The listing builds one solid part. Answer for the finished solid, in the listing's coordinates (mm). A direction names the side the tool comes from. Give positions to 0.01 mm unless a question says otherwise; leave off trailing zeros. Order: outer loops, then holes, each group sorted by start corner. A loop starts at its lowest first (then second) coordinate and runs counter-clockwise, first axis right, second up.
```python
from build123d import *

# Parameters (mm, degrees)
SKETCH_1_R          = 54
SKETCH_1_R_2        = 3
EXTRUDE_1_DEPTH     = 5
SKETCH_3_R          = 4
CUT_EXTRUDE_2_DEPTH = 77.531039455
SKETCH_4_R          = 2
EXTRUDE_2_DEPTH     = 12
CUT_EXTRUDE_START   = -3.2
SKETCH_6_R          = 2
SKETCH_6_R_2        = 1.8
CUT_EXTRUDE_3_DEPTH = 0.5
SKETCH_7_R          = 4
EXTRUDE_3_DEPTH     = 2
CHAMFER_1_SIZE      = 1
CUT_EXTRUDE_START_2 = -0.5
SKETCH_9_W          = 2
SKETCH_9_H          = 2
CUT_EXTRUDE_5_DEPTH = 4
FILLET_1_R          = 0.1


with BuildPart() as part:
    # Sketch 1 → Extrude 1 (new body)
    with BuildSketch(Plane.XY):
        Circle(SKETCH_1_R)
        Circle(SKETCH_1_R_2, mode=Mode.SUBTRACT)
    extrude(amount=EXTRUDE_1_DEPTH)

    # Sketch 3 → Cut-Extrude 2 (cut, through all)
    with BuildSketch(Plane(origin=(0, 0, 0), x_dir=(-1, 0, 0), z_dir=(0, 0, -1))):
        with Locations((-5.091227954, 19.341132281)):
            Circle(SKETCH_3_R)
        with Locations((10.076203981, 17.276287603)):
            Circle(SKETCH_3_R)
        with Locations((19.341132281, 5.091227954)):
            Circle(SKETCH_3_R)
        with Locations((17.276287603, -10.076203981)):
            Circle(SKETCH_3_R)
        with Locations((5.091227954, -19.341132281)):
            Circle(SKETCH_3_R)
        with Locations((-10.076203981, -17.276287603)):
            Circle(SKETCH_3_R)
        with Locations((-19.341132281, -5.091227954)):
            Circle(SKETCH_3_R)
        with Locations((-17.276287603, 10.076203981)):
            Circle(SKETCH_3_R)
    extrude(amount=-CUT_EXTRUDE_2_DEPTH, mode=Mode.SUBTRACT)

    # Sketch 4 → Extrude 2 (add)
    with BuildSketch(Plane.XY.offset(5)):
        with Locations((2.976659474, 6.884003078)):
            Circle(SKETCH_4_R)
        with Locations((9.178670771, -3.968879298)):
            Circle(SKETCH_4_R)
    extrude(amount=EXTRUDE_2_DEPTH)

    # Sketch 6 → Cut-Extrude 3 (cut)
    with BuildSketch(Plane.XY.offset(17).offset(CUT_EXTRUDE_START)):
        with Locations((2.976659474, 6.884003078)):
            Circle(SKETCH_6_R)
        with Locations((2.976659474, 6.884003078)):
            Circle(SKETCH_6_R_2, mode=Mode.SUBTRACT)
    extrude(amount=CUT_EXTRUDE_3_DEPTH, mode=Mode.SUBTRACT)

    # Sketch 7 → Extrude 3 (add)
    with BuildSketch(Plane.XY.offset(17)):
        with Locations((9.178670771, -3.968879298)):
            Circle(SKETCH_7_R)
    extrude(amount=-EXTRUDE_3_DEPTH)

    # Chamfer 1
    chamfer_1_edges = [part.edges().sort_by_distance(p)[0] for p in [
        (0.976659474, 6.884003078, 5),
        (7.178670771, -3.968879298, 5),
    ]]
    chamfer(chamfer_1_edges, length=CHAMFER_1_SIZE)

    # Sketch 9 → Cut-Extrude 5 (cut)
    with BuildSketch(Plane.XY.offset(5).offset(CUT_EXTRUDE_START_2)):
        with Locations((0, -3)):
            Rectangle(SKETCH_9_W, SKETCH_9_H)
    extrude(amount=-CUT_EXTRUDE_5_DEPTH, mode=Mode.SUBTRACT)

    # Fillet 1
    fillet_1_edges = [part.edges().sort_by_distance(p)[0] for p in [
        (1, -4, 2.5),
        (-1, -4, 2.5),
    ]]
    fillet(fillet_1_edges, radius=FILLET_1_R)


solid = part.part
```
1) Find section B-B (z = 10.5). Write down the section's boundary in (x, y).
Geometry says:
outline: circle Ø4 at (2.98, 6.88); circle Ø4 at (9.18, -3.97)
2) Given P1, Ø8, axis at y = 16.5, z = 14.5, coming from the +X side; P2, Ø13, axis at x = -17.28, y = -10.08, coming from the +Z side; P3, Ø10, axis at y = -26.5, z = 4, coming from the -X side; P4, Ø0.5, axis at y = -3.5, z = 3.5, coming from the +X side, each flat-ended and moving along its own axis, determine where each tip first touches the part or whether it passes through.
Geometry says:
P1: passes through
P2: stops at z = 5
P3: stops at x = -49.54
P4: stops at x = 53.9
3) Find section A-A (z = 2.5). Count the separate pieces of the cut face and the enclosed holes in it, then the cut area to 3 significant figures.
Geometry says:
separate pieces: 1
enclosed holes: 9
area: 8,730 mm2
4) Find section D-D (y = -35). Write down the section's boundary in (x, z), then the cut area to 3 significant figures.
Geometry says:
outline: (-41.12, 0) - (41.12, 0) - (41.12, 5) - (-41.12, 5) - close
area: 411 mm2
5) A tool of negligible diameter and unlimited length cuts with its end or side. For faces 4 (the cylindrical face through (4.05, 8.57, 15.63)), 5 (the flat face through (9, -4, 17)), 6 (the cylindrical face through (7.18, -3.88, 10.44)), from which of +Z, -Z, +X, -X, +Y, -Y can it reach the whole face along a straight path? Write none if from no direction.
Geometry says:
face 4: +Z
face 5: +Z, +X, -X, +Y, -Y
face 6: none
6) For a pull along Y with two mould halves and no side action, classify faces 1 (the flat face through (7, -5, 15)), 2 (the cylindrical face through (-11.706, -52.716, 2.465)), 3 (the cylindrical face through (5.612, 23.307, 2.465)) as +Y half, -Y half, draft (parallel to the pull), parting line (faces both ways), or undercut.
Geometry says:
face 1: draft
face 2: parting line
face 3: undercut
7) Find section C-C (x = 39.5). Write down the section's boundary in (y, z), then the cut area to 3 significant figures.
Geometry says:
outline: (-36.82, 0) - (36.82, 0) - (36.82, 5) - (-36.82, 5) - close
area: 368 mm2
8) Straight lines are drawn through the part: probe 1 along X at (y, z) = (16.5, 1); probe 2 along Z at (x, y) = (34, -15); probe 3 along Y at (x, z) = (5, 2.25). For each, find the intervals that lie inside material, in ascending order.
Geometry says:
probe 1: x = -51.42 to -14, -6.15 to 2.28, 7.91 to 51.42
probe 2: z = 0 to 5
probe 3: y = -53.77 to 15.34, 23.34 to 53.77
